```python
from build123d import *

# Parameters (mm, degrees)
BOX027_W     = 26
BOX027_H     = 33.6
BOX027_DEPTH = 1.7
BOX026_W     = 26.1
BOX026_H     = 32.2
BOX026_DEPTH = 6.7
BOX025_W     = 27.5
BOX025_H     = 36.6
BOX025_DEPTH = 8.2
FILLET001_R  = 1


with BuildPart() as pcb_extract_cube001:
    # Box027 → Box027 (new body)
    with BuildSketch(Plane(origin=(1.5, 1.5, 4.5), x_dir=(1, 0, 0), z_dir=(0, 0, 1))):
        with Locations((13, 16.8)):
            Rectangle(BOX027_W, BOX027_H)
    extrude(amount=BOX027_DEPTH)


with BuildPart() as extract_fusion001:
    # Box026 → Box026 (new body)
    with BuildSketch(Plane(origin=(2.2, 2.2, 1.5), x_dir=(1, 0, 0), z_dir=(0, 0, 1))):
        with Locations((13.05, 16.1)):
            Rectangle(BOX026_W, BOX026_H)
    extrude(amount=BOX026_DEPTH)

    # Fusion003: union pcb extract cube001
    add(pcb_extract_cube001.part)


with BuildPart() as lion_manager_cut:
    # Box025 → Box025 (new body)
    with BuildSketch(Plane.XY):
        with Locations((13.75, 18.3)):
            Rectangle(BOX025_W, BOX025_H)
    extrude(amount=BOX025_DEPTH)

    # Fillet001
    fillet001_edges = [lion_manager_cut.edges().sort_by_distance(p)[0] for p in [
        (0, 0, 4.1),
        (0, 36.6, 4.1),
        (27.5, 0, 4.1),
        (27.5, 36.6, 4.1),
    ]]
    fillet(fillet001_edges, radius=FILLET001_R)

    # Cut002: cut extract fusion001
    add(extract_fusion001.part, mode=Mode.SUBTRACT)


with BuildPart() as lion_manager_cut_1:
    # Cut002 placement: moved
    add(lion_manager_cut.part.moved(Location((-26, -1, -1))))


solid = lion_manager_cut_1.part
```
For this review, take the finished solid that the model builds, in its own axes (mm). A direction names the side the tool comes from. Round coordinates to 2 decimals unless told otherwise and drop trailing zeros. Loops run counter-clockwise (first coordinate to the right, second up) from the corner with the lowest first, then second, coordinate; pieces in that order, holes last.
Q1. Insertion check: pin 1 Ø2 at (y, z) = (17.5, 4) entering from +X; pin 2 Ø0.8 at (y, z) = (24, 4.5) entering from +X; pin 3 Ø8 at (x, y) = (-13.5, 11) entering from +Z. Each pin has a flat end and moves straight along its axis. Give the tip position at first contact, or say it passes through.
Result sheet:
pin 1: stops at x = -23.8
pin 2: stops at x = -24.5
pin 3: stops at z = 0.5
Q2. Mouldability with a two-part tool opening along Y and no side actions: class faces 1 (the face through (-12, 35.6, 3)), 2 (the face through (-25, 16, 7.2)), 3 (the face through (-11, 33.4, 6)) as +Y half, -Y half, draft (parallel to the pull), parting line (faces both ways), or undercut.
Result sheet:
face 1: +Y half
face 2: draft
face 3: undercut
Q3. Add section D-D on z = 4. Write out the cut boundary in (x, y).
Result sheet:
outline: (-26, 0) arc R1 ccw to (-25, -1) - (0.5, -1) arc R1 ccw to (1.5, 0) - (1.5, 0.5) - (-24.5, 0.5) - (-24.5, 34.1) - (1.5, 34.1) - (1.5, 34.6) arc R1 ccw to (0.5, 35.6) - (-25, 35.6) arc R1 ccw to (-26, 34.6) - close
Q4. To check wall thickness, follow line 1 along Y through (x, z) = (-12, 4.75); line 2 along Y through (x, z) = (-21.5, 3); line 3 along Z through (x, y) = (-18.25, 4). State the ranges of each line that lie inside material, in increasing order.
Result sheet:
line 1: y = -1 to 0.5, 34.1 to 35.6
line 2: y = -1 to 1.2, 33.4 to 35.6
line 3: z = -1 to 0.5
Q5. Machinability: for faces 4 (the face through (-12, 18, -1)), 5 (the face through (-11, 18, 0.5)), 6 (the face through (-24, 25, 3.5)), which of the approach directions +Z, -Z, +X, -X, +Y, -Y give a long, thin tool a straight path to every point of the face, cutting with its end or side? Answer none if there is none.
Result sheet:
face 4: -Z, +X, -X, +Y, -Y
face 5: +Z, +X
face 6: +X
Q6. Add section B-B on z = 6.75. Write out the cut boundary in (x, y), plus the area to 3 significant figures.
Result sheet:
outline: (-26, 0) arc R1 ccw to (-25, -1) - (0.5, -1) arc R1 ccw to (1.5, 0) - (1.5, 1.2) - (-23.8, 1.2) - (-23.8, 33.4) - (1.5, 33.4) - (1.5, 34.6) arc R1 ccw to (0.5, 35.6) - (-25, 35.6) arc R1 ccw to (-26, 34.6) - close
area: 191 mm2
Q7. Add section A-A on x = -4.75. Write out the cut boundary in (y, z).
Result sheet:
outline: (-1, -1) - (35.6, -1) - (35.6, 7.2) - (33.4, 7.2) - (33.4, 5.2) - (34.1, 5.2) - (34.1, 3.5) - (33.4, 3.5) - (33.4, 0.5) - (1.2, 0.5) - (1.2, 3.5) - (0.5, 3.5) - (0.5, 5.2) - (1.2, 5.2) - (1.2, 7.2) - (-1, 7.2) - close
Q8. Add section C-C on y = 7. Write out the cut boundary in (x, z), plus the area to 3 significant figures.
Result sheet:
outline: (-26, -1) - (1.5, -1) - (1.5, 0.5) - (-23.8, 0.5) - (-23.8, 3.5) - (-24.5, 3.5) - (-24.5, 5.2) - (-23.8, 5.2) - (-23.8, 7.2) - (-26, 7.2) - close
area: 54.8 mm2
